Could you check a few things on this model? Use its own coordinates, in mm. A direction names the side the tool comes from. Round coordinates to 2 decimals unless told otherwise and drop trailing zeros. Loops run counter-clockwise (first coordinate to the right, second up) from the corner with the lowest first, then second, coordinate; pieces in that order, holes last. Notation, with made-up numbers: M 57.25,42 L 76.25,42 A17 cw 76.25,64 Z; hole C 3,22.25 d8. An arc over 180 degrees is marked long. Answer in a Markdown table with one row per item.
```python
from build123d import *

# Parameters (mm, degrees)
BOSS_EXTRUDE2_DEPTH = 6.35
CUT_EXTRUDE1_DEPTH  = 7.3500001
BOSS_EXTRUDE3_DEPTH = 6.35
SKETCH10_R          = 3.96875
CUT_EXTRUDE2_DEPTH  = 7.35
SKETCH11_R          = 4.5
CUT_EXTRUDE4_DEPTH  = 7.35
BOSS_EXTRUDE4_DEPTH = 6.35
SKETCH13_R          = 1.75
CUT_EXTRUDE5_DEPTH  = 7.35
LPATTERN1_COUNT     = 2
LPATTERN1_PITCH     = 64
SKETCH15_R          = 1.75
CUT_EXTRUDE7_DEPTH  = 7.35
SKETCH16_R          = 1.75
CUT_EXTRUDE8_DEPTH  = 7.35
SKETCH17_R          = 1.75
CUT_EXTRUDE9_DEPTH  = 7.35
SKETCH18_R          = 1.75
SKETCH18_R_2        = 6.35
CUT_EXTRUDE10_DEPTH = 7.35
SKETCH19_R          = 3.96875
CUT_EXTRUDE11_DEPTH = 7.35
SKETCH20_R          = 3.96875
CUT_EXTRUDE12_DEPTH = 7.35
SKETCH21_R          = 5.677654576
BOSS_EXTRUDE5_DEPTH = 6.35
CUT_EXTRUDE13_DEPTH = 7.35
SKETCH23_R          = 1.75
CUT_EXTRUDE14_DEPTH = 7.35
FILLET1_R           = 3.175


with BuildPart() as part:
    # Sketch6 → Boss-Extrude2 (new body)
    with BuildSketch(Plane.XY):
        with BuildLine():
            Line((-68.006850091, -76.67090114), (-109.486767671, -48.656527855))
            Line((-109.486767671, -48.656527855), (-118.371760678, -61.812230963))
            Line((-118.371760678, -61.812230963), (18.447551645, -154.216158235))
            Line((18.447551645, -154.216158235), (135.729459338, 19.43912279))
            Line((135.729459338, 19.43912279), (-1.089852986, 111.843050063))
            Line((-1.089852986, 111.843050063), (-73.946795643, 3.966284577))
            Line((-73.946795643, 3.966284577), (-56.624438948, -7.732749433))
            ThreePointArc((-56.624438948, -7.732749433), (-43.058385537, 37.577891571), (0, 57.15))
            ThreePointArc((0, 57.15), (56.404848571, 31.095576642), (70.829334649, -29.338471048))
            add(Edge.make_bspline(
                [(70.829334649, -29.338471048), (70.811686062, -29.418295928), (70.776015112, -29.578104383), (70.713320217, -29.85478305), (70.619021771, -30.262929245), (70.501052001, -30.762086912), (70.364034474, -31.322191481), (70.199318515, -31.970958926), (70.000453855, -32.723919765), (69.795103485, -33.469783355), (69.582015398, -34.214296028), (69.361377803, -34.956693289), (69.133257682, -35.696762218), (68.838782679, -36.61892651), (68.470566207, -37.720710028), (68.019498024, -38.998776477), (67.474836154, -40.448808619), (66.901337925, -41.887676852), (66.299328392, -43.31485223), (65.669141732, -44.729810424), (65.011119088, -46.132040323), (64.325609411, -47.52103904), (63.612968547, -48.896314904), (62.87355937, -50.257385735), (62.107751613, -51.603779381), (61.315921169, -52.935034173), (60.49845004, -54.250698756), (59.655726138, -55.550331897), (58.571247582, -57.154294757), (57.220953058, -59.045283389), (55.576035723, -61.200397094), (53.604026134, -63.590264702), (51.54329346, -65.904053004), (49.39728314, -68.138962994), (47.169496434, -70.29235602), (44.863486103, -72.361752995), (42.482847363, -74.344831806), (40.031215607, -76.239428526), (36.882516177, -78.494556171), (32.976808929, -81.016011003), (28.250788286, -83.68089187), (21.41551215, -86.919136497), (14.30829026, -89.526654921), (6.996956895, -91.488176442), (-0.451922312, -92.797413176), (-6.61686174, -93.456358442), (-12.81195397, -93.702029749), (-19.009644204, -93.537285056), (-25.183124422, -92.966685286), (-31.306438312, -91.996382122), (-36.598524037, -90.804323442), (-41.072542301, -89.543185606), (-44.752319298, -88.33589156), (-47.664184976, -87.27761875), (-50.541347258, -86.128353728), (-53.381128552, -84.889612663), (-56.180924218, -83.562977818), (-58.593536599, -82.326710176), (-60.633378351, -81.214215821), (-62.313751085, -80.252471782), (-63.646071553, -79.462491566), (-64.966093336, -78.652178853), (-66.222359154, -77.854259082), (-67.143044791, -77.250601571), (-67.736251212, -76.85365602), (-68.006850091, -76.67090114)],
                knots=[0.071020771, 0.071020771, 0.071020771, 0.071020771, 0.071020771, 0.072848477, 0.074676184, 0.07650389, 0.078331597, 0.08198701, 0.085642423, 0.089297836, 0.092953249, 0.096608662, 0.100264075, 0.103919488, 0.107574901, 0.114885727, 0.122196554, 0.12950738, 0.136818214, 0.144129048, 0.151439882, 0.158750716, 0.166061558, 0.173372401, 0.180683243, 0.187994085, 0.195304924, 0.202615763, 0.209926602, 0.217237441, 0.231859103, 0.246480766, 0.261102426, 0.275724085, 0.290345754, 0.304967424, 0.319589099, 0.334210774, 0.348832457, 0.36345414, 0.392697464, 0.421940789, 0.451184112, 0.506140643, 0.535383973, 0.564627303, 0.593870641, 0.623113979, 0.652357319, 0.68160066, 0.710843985, 0.740087309, 0.754708984, 0.769330659, 0.783952333, 0.798574008, 0.813195669, 0.82781733, 0.842438991, 0.849749821, 0.857060652, 0.86437149, 0.871682327, 0.878993165, 0.885158103, 0.885158103, 0.885158103, 0.885158103, 0.885158103], degree=4))
        make_face()
    extrude(amount=BOSS_EXTRUDE2_DEPTH)

    # Sketch8 → Cut-Extrude1 (cut, through all)
    with BuildSketch(Plane.XY.offset(6.35)):
        Polygon((-71.011229489, -93.798205788), (-53.378672597, -90.381637707), (-42.854110111, -97.489632113), (-39.43754203, -115.122189004), align=None)
    extrude(amount=-CUT_EXTRUDE1_DEPTH, mode=Mode.SUBTRACT)

    # Sketch9 → Boss-Extrude3 (add, through all)
    with BuildSketch(Plane.XY.offset(6.35)):
        Polygon((-1.089852986, 111.843050063), (-109.486767671, -48.656527855), (27.332544652, -141.060455127), (135.729459338, 19.43912279), align=None)
    extrude(amount=-BOSS_EXTRUDE3_DEPTH)

    # Sketch10 → Cut-Extrude2 (cut, through all)
    with BuildSketch(Plane.XY.offset(6.35)):
        with Locations((4.996496209, -84.796642912)):
            Circle(SKETCH10_R)
        with Locations((40.816310536, -31.759477627)):
            Circle(SKETCH10_R)
        with Locations((76.636124864, 21.277687659)):
            Circle(SKETCH10_R)
        with Locations((-45.295165913, -45.214466102)):
            Circle(SKETCH10_R)
    extrude(amount=-CUT_EXTRUDE2_DEPTH, mode=Mode.SUBTRACT)

    # Sketch11 → Cut-Extrude4 (cut, through all)
    with BuildSketch(Plane.XY.offset(6.35)):
        Circle(SKETCH11_R)
    extrude(amount=-CUT_EXTRUDE4_DEPTH, mode=Mode.SUBTRACT)

    # Sketch12 → Boss-Extrude4 (add, through all)
    with BuildSketch(Plane.XY.offset(6.35)):
        Polygon((135.729459338, 19.43912279), (67.319803176, 65.641086427), (88.643786393, 97.214773886), (157.053442554, 51.01281025), align=None)
    extrude(amount=-BOSS_EXTRUDE4_DEPTH)

    # Sketch13 → Cut-Extrude5 (cut, through all)
    with BuildSketch(Plane.XY.offset(6.35)):
        with Locations((94.899221836, -29.671127724)):
            Circle(SKETCH13_R)
    cut_extrude5 = extrude(amount=-CUT_EXTRUDE5_DEPTH, mode=Mode.SUBTRACT)

    # LPattern1: Cut-Extrude5 ×2
    with Locations(*[Vector(-0.559684599, -0.828705708, 0) * (i * LPATTERN1_PITCH) for i in range(1, LPATTERN1_COUNT)]):
        add(cut_extrude5, mode=Mode.SUBTRACT)

    # Sketch15 → Cut-Extrude7 (cut, through all)
    with BuildSketch(Plane.XY.offset(6.35)):
        with Locations((-105.147343009, -59.249804902)):
            Circle(SKETCH15_R)
        with Locations((15.885125585, -140.991740566)):
            Circle(SKETCH15_R)
        with Locations((1.472573075, 98.618632394)):
            Circle(SKETCH15_R)
    extrude(amount=-CUT_EXTRUDE7_DEPTH, mode=Mode.SUBTRACT)

    # Sketch16 → Cut-Extrude8 (cut, through all)
    with BuildSketch(Plane.XY.offset(6.35)):
        with Locations((92.060354474, 79.582216994)):
            Circle(SKETCH16_R)
        with Locations((139.420885662, 47.596242169)):
            Circle(SKETCH16_R)
    extrude(amount=-CUT_EXTRUDE8_DEPTH, mode=Mode.SUBTRACT)

    # Sketch17 → Cut-Extrude9 (cut, through all)
    with BuildSketch(Plane.XY.offset(6.35)):
        with Locations((-26.311406216, 17.769986014)):
            Circle(SKETCH17_R)
        with Locations((17.769986014, 26.311406216)):
            Circle(SKETCH17_R)
    extrude(amount=-CUT_EXTRUDE9_DEPTH, mode=Mode.SUBTRACT)

    # Sketch18 → Cut-Extrude10 (cut, through all)
    with BuildSketch(Plane.XY.offset(6.35)):
        with Locations((75.468896753, 66.798604333)):
            Circle(SKETCH18_R)
        with Locations((74.378499235, 51.337005669)):
            Circle(SKETCH18_R)
        with Locations((87.223437703, 42.661894386)):
            Circle(SKETCH18_R)
        with Locations((101.158773688, 49.448381768)):
            Circle(SKETCH18_R)
        with Locations((102.249171205, 64.909980432)):
            Circle(SKETCH18_R)
        with Locations((89.404232738, 73.585091715)):
            Circle(SKETCH18_R)
        with Locations((99.589076537, 21.914747078)):
            Circle(SKETCH18_R)
        with Locations((104.266720973, 36.692082512)):
            Circle(SKETCH18_R)
        with Locations((119.403091077, 40.029791318)):
            Circle(SKETCH18_R)
        with Locations((129.861816745, 28.59016469)):
            Circle(SKETCH18_R)
        with Locations((125.18417231, 13.812829255)):
            Circle(SKETCH18_R)
        with Locations((110.047802206, 10.47512045)):
            Circle(SKETCH18_R)
        with Locations((105.180381325, -7.122099496)):
            Circle(SKETCH18_R)
        with Locations((96.077150237, 5.423066257)):
            Circle(SKETCH18_R)
        with Locations((80.661102457, 3.812019754)):
            Circle(SKETCH18_R)
        with Locations((74.348285765, -10.344192501)):
            Circle(SKETCH18_R)
        with Locations((83.451516853, -22.889358254)):
            Circle(SKETCH18_R)
        with Locations((98.867564633, -21.278311751)):
            Circle(SKETCH18_R)
        with Locations((84.396043028, 52.322553097)):
            Circle(SKETCH18_R_2)
        with Locations((108.051811284, 27.364940468)):
            Circle(SKETCH18_R_2)
        with Locations((95.429892272, -4.622009378)):
            Circle(SKETCH18_R_2)
    extrude(amount=-CUT_EXTRUDE10_DEPTH, mode=Mode.SUBTRACT)

    # Sketch19 → Cut-Extrude11 (cut, through all)
    with BuildSketch(Plane.XY.offset(6.35)):
        with Locations((-65.680233685, -85.904783923)):
            Circle(SKETCH19_R)
    extrude(amount=-CUT_EXTRUDE11_DEPTH, mode=Mode.SUBTRACT)

    # Sketch20 → Cut-Extrude12 (cut, through all)
    with BuildSketch(Plane.XY.offset(6.35)):
        with Locations((-105.147343009, -59.249804902)):
            Circle(SKETCH20_R)
    extrude(amount=-CUT_EXTRUDE12_DEPTH, mode=Mode.SUBTRACT)

    # Sketch21 → Boss-Extrude5 (add, through all)
    with BuildSketch(Plane.XY.offset(6.35)):
        with Locations((-65.680233685, -85.904783923)):
            Circle(SKETCH21_R)
    extrude(amount=-BOSS_EXTRUDE5_DEPTH)

    # Sketch22 → Cut-Extrude13 (cut, through all)
    with BuildSketch(Plane.XY.offset(6.35)):
        Polygon((85.800588631, 93.004948891), (87.167215863, 85.951926135), (71.529628171, 62.797888664), (67.319803176, 65.641086427), align=None)
    extrude(amount=-CUT_EXTRUDE13_DEPTH, mode=Mode.SUBTRACT)

    # Sketch23 → Cut-Extrude14 (cut, through all)
    with BuildSketch(Plane(origin=(0, 0, 0), x_dir=(-1, 0, 0), z_dir=(0, 0, -1))):
        with Locations((-8.248274978, 59.561032446)):
            Circle(SKETCH23_R)
        with Locations((18.270307664, 77.470939609)):
            Circle(SKETCH23_R)
    extrude(amount=-CUT_EXTRUDE14_DEPTH, mode=Mode.SUBTRACT)

    # Fillet1
    fillet1_edges = [part.edges().sort_by_distance(p)[0] for p in [
        (-1.089852986, 111.843050063, 3.175),
        (18.447551645, -154.216158235, 3.175),
        (-118.371760678, -61.812230963, 3.175),
        (87.167215863, 85.951926135, 3.175),
        (85.800588631, 93.004948891, 3.175),
        (71.529628171, 62.797888664, 3.175),
        (-39.43754203, -115.122189004, 3.175),
        (-71.011229489, -93.798205788, 3.175),
        (-53.378672597, -90.381637707, 3.175),
        (-42.854110111, -97.489632113, 3.175),
        (157.053442554, 51.01281025, 3.175),
        (88.643786393, 97.214773886, 3.175),
    ]]
    fillet(fillet1_edges, radius=FILLET1_R)


solid = part.part
```
1) If we mould it in two halves opening along X, with no side actions, what happens to faces 3 (the face through (-11.645, -133.893, 3.131)), 4 (the face through (21, -19, 6.35)), 5 (the face through (-43.16, -41.87, 3.22))? For each: released by +X, released by -X, zero draft, split by the parting line, or undercut.
Computed:
| item | result |
|---|---|
| face 3 | released by -X |
| face 4 | zero draft |
| face 5 | undercut |
2) I want a section at B-B, the plane y = -70. Please give me the cut outline in (x, z).
Computed:
| item | result |
|---|---|
| outline | M -106.25,0 L 75.32,0 L 75.32,6.35 L -106.25,6.35 Z |
3) I want a section at A-A, the plane z = 4.5. State how many separate pieces and enclosed holes the cut face has, plus the area to 3 significant figures.
Computed:
| item | result |
|---|---|
| separate pieces | 1 |
| enclosed holes | 36 |
| area | 36,300 mm² |
4) Which directions (+Z, -Z, +X, -X, +Y, -Y) give clear straight access to the entire face, cutting with the end or side of a thin tool? Please do faces 1 (the face through (-62.3, -92.11, 3.22)), 2 (the face through (98.844, 0.732, 3.219)).
Computed:
| item | result |
|---|---|
| face 1 | +Z, -Z, -Y |
| face 2 | +Z, -Z |
5) Will these pins go through, and if not, where does the flat tip stop? P1, Ø2, axis at x = -53.5, z = 2.5, coming from the +Y side; P2, Ø1.5, axis at x = 50, z = 1, coming from the -Y side; P3, Ø1, axis at y = -9.5, z = 2, coming from the -X side.
Computed:
| item | result |
|---|---|
| P1 | stops at y = 35.72 |
| P2 | stops at y = -108.61 |
| P3 | stops at x = -83.38 |
6) I need wall thicknesses on line 1 (Y direction, x = 81, z = 2.25); line 2 (X direction, y = -4, z = 4); line 3 (Y direction, x = 74, z = 5). Which ranges of each line are inside material? Lowest first, please.
Computed:
| item | result |
|---|---|
| line 1 | y = -61.6 to 2.1, 5.53 to 46.96, 57.69 to 76.82 |
| line 2 | x = -79.33 to -2.06, 2.06 to 89.11, 101.75 to 119.9 |
| line 3 | y = -71.96 to -12.06, -8.63 to 18.31, 24.24 to 49.63, 53.05 to 65.85 |
